For this review, take the finished solid that the model builds, in its own axes (mm). A direction names the side the tool comes from. Round coordinates to 2 decimals unless told otherwise and drop trailing zeros. Loops run counter-clockwise (first coordinate to the right, second up) from the corner with the lowest first, then second, coordinate; pieces in that order, holes last. Notation, with made-up numbers: (7.25, -39) -> (34.25, -39) arc R37 cw to (34.25, 0) -> close; hole circle Ø11 at (-33.75, -18). An arc over 180 degrees is marked (long way). Write each question's results on one line, items separated by ' | '.
```python
from build123d import *

# Parameters (mm, degrees)
F1_DEPTH      = 76.2
F2_W          = 304.8
F2_H          = 76.2
F3_DEPTH      = 304.8
F3_DEPTH_BACK = 127


with BuildPart() as f1:
    # F0 (on Front) → F1 (new body)
    with BuildSketch(Plane.XZ):
        Polygon((-152.4, 38.1), (-152.4, -38.1), (152.4, -38.1), (152.4, 38.1), (-101.6, 38.1), (-101.6, 444.5), (-152.4, 444.5), align=None)
    extrude(amount=F1_DEPTH)

    # F2 (on face) → F3 (join, two sides)
    with BuildSketch(Plane(origin=(0, 0, 0), x_dir=(-1, 0, 0), z_dir=(0, 1, 0))) as f3_sk:
        Rectangle(F2_W, F2_H)
    extrude(amount=F3_DEPTH)
    extrude(f3_sk.sketch, amount=-F3_DEPTH_BACK)


solid = f1.part
```
1. For pin 1 (1.5 mm diameter, centred on x = 98.5, y = -62.5, fed in from +Z); pin 2 (23 mm diameter, centred on y = -27, z = 212.5, fed in from +X), all flat-tipped, find the tip position at first contact; note any pin that passes through.
Values found:
pin 1: stops at z = 38.1 | pin 2: stops at x = -101.6
2. Consider section A-A (y = 91). State the section outline as (x, z) points.
Values found:
outline: (-152.4, -38.1) -> (152.4, -38.1) -> (152.4, 38.1) -> (-152.4, 38.1) -> close
3. Consider section C-C (y = -32). State the section outline as (x, z) points.
Values found:
outline: (-152.4, -38.1) -> (152.4, -38.1) -> (152.4, 38.1) -> (-101.6, 38.1) -> (-101.6, 444.5) -> (-152.4, 444.5) -> close
4. Consider section B-B (z = 128). State the section outline as (x, y) points, plus the area to 3 significant figures.
Values found:
outline: (-152.4, -76.2) -> (-101.6, -76.2) -> (-101.6, 0) -> (-152.4, 0) -> close | area: 3,870 mm2
5. To check wall thickness, follow probe 1 along Y at (x, z) = (-128.5, 147); probe 2 along Z at (x, y) = (96.5, -55.5); probe 3 along X at (y, z) = (-18.5, 188). State the ranges of each line that lie inside material, in increasing order.
Values found:
probe 1: y = -76.2 to 0 | probe 2: z = -38.1 to 38.1 | probe 3: x = -152.4 to -101.6
6. Draft analysis for pull direction Z (two halves, no side actions). For faces 4 (the face through (2, 304.8, 1)), 5 (the face through (2, 92, -38.1)), 6 (the face through (-127, -38, 444.5)), state which applies: released by +Z, released by -Z, zero draft, split by the parting line, or undercut.
Values found:
face 4: zero draft | face 5: released by -Z | face 6: released by +Z
7. Tool access review of faces 1 (the face through (-101.6, -38, 238)), 2 (the face through (-127, 0, 244)), 3 (the face through (-127, -76.2, 244)): name each direction out of +Z, -Z, +X, -X, +Y, -Y from which nothing blocks a thin tool from reaching the whole face with its end or side.
Values found:
face 1: +Z, +X, +Y, -Y | face 2: +Z, +X, -X, +Y | face 3: +Z, +X, -X, -Y
